Autodesk Inventor part; units mm, degrees
ref_plane "pins_to_body_XY" through (0, 0, 0) normal (0, -1, 0) x (1, 0, 0)
ref_plane "pins_to_body_YZ" through (0, 0, 0) normal (1, 0, 0) x (0, 0, 1)
ref_plane "pins_to_body_ZX" through (0, 0, 0) normal (0, 0, 1) x (0, -1, 0)
sketch "Sketch_1" plane through (0, 0, 0) normal (0, 1, 0) x (-1, 0, 0)
  line L0 (7.0485, -7.0485) -> (7.0485, 7.0485)
  line L1 (7.0485, 7.0485) -> (-7.0485, 7.0485)
  line L2 (-7.0485, 7.0485) -> (-7.0485, -7.0485)
  line L3 (-7.0485, -7.0485) -> (7.0485, -7.0485)
extrude "Extrusion1" add sketch "Sketch_1" along normal blind 0.0254
sketch "Sketch_3" plane through (0, 0, 7.0485) normal (0, 0, 1) x (1, 0, 0)
  line L0 (-0.7112, 0.0254) -> (-0.7112, -0.7366)
  line L1 (-0.7112, -0.7366) -> (-0.5842, -0.7366)
  line L2 (-0.5842, -0.7366) -> (-0.5842, -3.048)
  line L3 (-0.5842, -3.048) -> (-0.4318, -3.048)
  line L4 (-0.4318, -3.048) -> (-0.4318, -3.556)
  line L5 (-0.4318, -3.556) -> (-0.5842, -3.556)
  line L6 (-0.5842, -3.556) -> (-0.5842, -5.08)
  arc A0 (-0.5842, -5.08) -> (0.5842, -5.08) centre (0, -4.772) ccw
  line L7 (0.5842, -5.08) -> (0.5842, -3.556)
  line L8 (0.5842, -3.556) -> (0.4318, -3.556)
  line L9 (0.4318, -3.556) -> (0.4318, -3.048)
  line L10 (0.4318, -3.048) -> (0.5842, -3.048)
  line L11 (0.5842, -3.048) -> (0.5842, -0.7366)
  line L12 (0.5842, -0.7366) -> (0.7112, -0.7366)
  line L13 (0.7112, -0.7366) -> (0.7112, 0.0254)
  line L14 (0.7112, 0.0254) -> (-0.7112, 0.0254)
extrude "Extrusion2" add sketch "Sketch_3" against normal blind 0.6096
sketch "Sketch_5" plane through (0, 0, 0) normal (0, 0, 1) x (1, 0, 0)
  line L0 (4.0005, 0.0254) -> (4.0005, -3.2512)
  arc A0 (4.0005, -3.2512) -> (4.2545, -3.5052) centre (4.2545, -3.2512) ccw
  line L1 (4.2545, -3.5052) -> (5.7531, -3.5052)
  arc A1 (5.7531, -3.5052) -> (6.0071, -3.2512) centre (5.7531, -3.2512) ccw
  line L2 (6.0071, -3.2512) -> (6.0071, 0.0254)
  line L3 (6.0071, 0.0254) -> (4.0005, 0.0254)
  arc A2 (4.4577, -2.3876) -> (5.5499, -2.3876) centre (5.0038, -0.8728) ccw
  line L4 (5.5499, -2.3876) -> (5.5499, -0.5842)
  arc A3 (5.5499, -0.5842) -> (4.4577, -0.5842) centre (5.0038, -1.9147) ccw
  line L5 (4.4577, -0.5842) -> (4.4577, -2.3876)
extrude "Extrusion3" add sketch "Sketch_5" along normal mid plane 0.7874
sketch "Sketch_6" plane through (0, 0, 0) normal (0, 0, 1) x (1, 0, 0)
  line L0 (-6.0071, 0.0254) -> (-6.0071, -3.2512)
  arc A0 (-6.0071, -3.2512) -> (-5.7531, -3.5052) centre (-5.7531, -3.2512) ccw
  line L1 (-5.7531, -3.5052) -> (-4.2545, -3.5052)
  arc A1 (-4.2545, -3.5052) -> (-4.0005, -3.2512) centre (-4.2545, -3.2512) ccw
  line L2 (-4.0005, -3.2512) -> (-4.0005, 0.0254)
  line L3 (-4.0005, 0.0254) -> (-6.0071, 0.0254)
  line L4 (-5.5499, -0.5842) -> (-5.5499, -2.3876)
  arc A2 (-5.5499, -2.3876) -> (-4.4577, -2.3876) centre (-5.0038, -0.8728) ccw
  line L5 (-4.4577, -2.3876) -> (-4.4577, -0.5842)
  arc A3 (-4.4577, -0.5842) -> (-5.5499, -0.5842) centre (-5.0038, -1.9147) ccw
extrude "Extrusion4" add sketch "Sketch_6" along normal mid plane 0.7874
sketch "Sketch_7" plane through (0, 0, -4.699) normal (0, 0, 1) x (1, 0, 0)
  line L0 (4.0005, 0.0254) -> (4.0005, -2.7432)
  arc A0 (4.0005, -2.7432) -> (4.2545, -2.9972) centre (4.2545, -2.7432) ccw
  line L1 (4.2545, -2.9972) -> (5.7531, -2.9972)
  arc A1 (5.7531, -2.9972) -> (6.0071, -2.7432) centre (5.7531, -2.7432) ccw
  line L2 (6.0071, -2.7432) -> (6.0071, 0.0254)
  line L3 (6.0071, 0.0254) -> (4.0005, 0.0254)
  arc A2 (4.4577, -2.1336) -> (5.5499, -2.1336) centre (5.0038, -0.6188) ccw
  line L4 (5.5499, -2.1336) -> (5.5499, -0.3302)
  arc A3 (5.5499, -0.3302) -> (4.4577, -0.3302) centre (5.0038, -1.6607) ccw
  line L5 (4.4577, -0.3302) -> (4.4577, -2.1336)
extrude "Extrusion5" add sketch "Sketch_7" along normal mid plane 0.7874
sketch "Sketch_8" plane through (0, 0, -4.699) normal (0, 0, 1) x (1, 0, 0)
  line L0 (-6.0071, 0.0254) -> (-6.0071, -2.7432)
  arc A0 (-6.0071, -2.7432) -> (-5.7531, -2.9972) centre (-5.7531, -2.7432) ccw
  line L1 (-5.7531, -2.9972) -> (-4.2545, -2.9972)
  arc A1 (-4.2545, -2.9972) -> (-4.0005, -2.7432) centre (-4.2545, -2.7432) ccw
  line L2 (-4.0005, -2.7432) -> (-4.0005, 0.0254)
  line L3 (-4.0005, 0.0254) -> (-6.0071, 0.0254)
  line L4 (-5.5499, -0.3302) -> (-5.5499, -2.1336)
  arc A2 (-5.5499, -2.1336) -> (-4.4577, -2.1336) centre (-5.0038, -0.6188) ccw
  line L5 (-4.4577, -2.1336) -> (-4.4577, -0.3302)
  arc A3 (-4.4577, -0.3302) -> (-5.5499, -0.3302) centre (-5.0038, -1.6607) ccw
extrude "Extrusion6" add sketch "Sketch_8" along normal mid plane 0.7874
sketch "Sketch_9" plane through (0, 0, 4.699) normal (0, 0, 1) x (1, 0, 0)
  line L0 (4.0005, 0.0254) -> (4.0005, -2.7432)
  arc A0 (4.0005, -2.7432) -> (4.2545, -2.9972) centre (4.2545, -2.7432) ccw
  line L1 (4.2545, -2.9972) -> (5.7531, -2.9972)
  arc A1 (5.7531, -2.9972) -> (6.0071, -2.7432) centre (5.7531, -2.7432) ccw
  line L2 (6.0071, -2.7432) -> (6.0071, 0.0254)
  line L3 (6.0071, 0.0254) -> (4.0005, 0.0254)
  arc A2 (4.4577, -2.1336) -> (5.5499, -2.1336) centre (5.0038, -0.6188) ccw
  line L4 (5.5499, -2.1336) -> (5.5499, -0.3302)
  arc A3 (5.5499, -0.3302) -> (4.4577, -0.3302) centre (5.0038, -1.6607) ccw
  line L5 (4.4577, -0.3302) -> (4.4577, -2.1336)
extrude "Extrusion7" add sketch "Sketch_9" along normal mid plane 0.7874
sketch "Sketch_10" plane through (0, 0, 4.699) normal (0, 0, 1) x (1, 0, 0)
  line L0 (-6.0071, 0.0254) -> (-6.0071, -2.7432)
  arc A0 (-6.0071, -2.7432) -> (-5.7531, -2.9972) centre (-5.7531, -2.7432) ccw
  line L1 (-5.7531, -2.9972) -> (-4.2545, -2.9972)
  arc A1 (-4.2545, -2.9972) -> (-4.0005, -2.7432) centre (-4.2545, -2.7432) ccw
  line L2 (-4.0005, -2.7432) -> (-4.0005, 0.0254)
  line L3 (-4.0005, 0.0254) -> (-6.0071, 0.0254)
  line L4 (-5.5499, -0.3302) -> (-5.5499, -2.1336)
  arc A2 (-5.5499, -2.1336) -> (-4.4577, -2.1336) centre (-5.0038, -0.6188) ccw
  line L5 (-4.4577, -2.1336) -> (-4.4577, -0.3302)
  arc A3 (-4.4577, -0.3302) -> (-5.5499, -0.3302) centre (-5.0038, -1.6607) ccw
extrude "Extrusion8" add sketch "Sketch_10" along normal mid plane 0.7874
sketch "Sketch_4" plane through (0, 0, -7.0485) normal (0, 0, 1) x (1, 0, 0)
  line L0 (-0.7112, 0.0254) -> (-0.7112, -0.7366)
  line L1 (-0.7112, -0.7366) -> (-0.5842, -0.7366)
  line L2 (-0.5842, -0.7366) -> (-0.5842, -3.048)
  line L3 (-0.5842, -3.048) -> (-0.4318, -3.048)
  line L4 (-0.4318, -3.048) -> (-0.4318, -3.556)
  line L5 (-0.4318, -3.556) -> (-0.5842, -3.556)
  line L6 (-0.5842, -3.556) -> (-0.5842, -5.08)
  arc A0 (-0.5842, -5.08) -> (0.5842, -5.08) centre (0, -4.772) ccw
  line L7 (0.5842, -5.08) -> (0.5842, -3.556)
  line L8 (0.5842, -3.556) -> (0.4318, -3.556)
  line L9 (0.4318, -3.556) -> (0.4318, -3.048)
  line L10 (0.4318, -3.048) -> (0.5842, -3.048)
  line L11 (0.5842, -3.048) -> (0.5842, -0.7366)
  line L12 (0.5842, -0.7366) -> (0.7112, -0.7366)
  line L13 (0.7112, -0.7366) -> (0.7112, 0.0254)
  line L14 (0.7112, 0.0254) -> (-0.7112, 0.0254)
extrude "Extrusion9" add sketch "Sketch_4" along normal blind 0.6096
ref_plane "pins_to_body_XY" through (0, 0, 0) normal (0, -1, 0) x (1, 0, 0)
ref_plane "pins_to_body_YZ" through (0, 0, 0) normal (1, 0, 0) x (0, 0, 1)
ref_plane "pins_to_body_ZX" through (0, 0, 0) normal (0, 0, 1) x (0, -1, 0)
properties part number "tlD-pins"
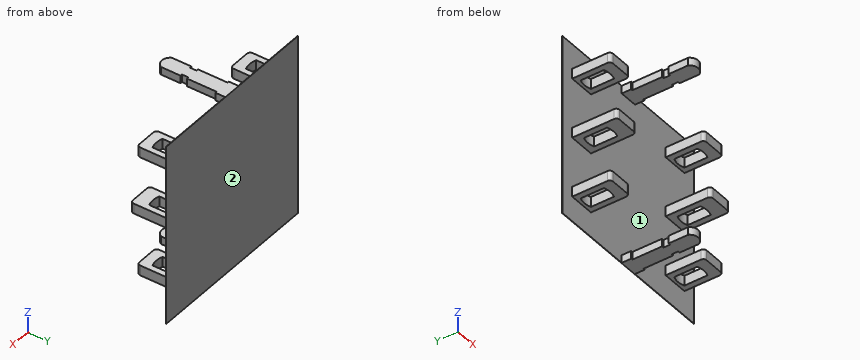
Part model, mm, in its own coordinate system. Face numbers are marked on the shaded views. Give positions to 0.01 mm unless a question says otherwise; leave off trailing zeros. Order: outer loops, then holes, each group sorted by start corner. A loop starts at its lowest first (then second) coordinate and runs counter-clockwise, first axis right, second up. Notation, with made-up numbers: M -12.5,22.5 L -0.5,22.5 A18 ccw -0.5,32.5 Z; hole C -1,33 d4. An arc over 180 degrees is marked long. Use a Markdown table: item, result. Add a question column.
(1) Saw through at A-A, the plane x = 4.75. Give the number of separate pieces and of enclosed holes in the cut face, and give its area (3 significant figures).
(2) Mould opens along Z. For the marked faces 1 and 2 say: +Z half, -Z half, draft (parallel to the pull), parting line (faces both ways), or undercut.
(3) Probe line 1 along X through (y, z) = (-3.75, 6.5); line 2 along X through (y, z) = (-2.8, -5). List the from-to ranges inside material, lowest first. Write a range as [from, to].
(4) Drop flat-ended pins along their axis: P1, Ø0.7, axis at y = -0.5, z = -6.5, coming from the -X side; P2, Ø3, axis at x = -3.5, y = -4.5, coming from the -Z side; P3, Ø1, axis at x = -0.5, z = -5, coming from the -Y side. Give the stop position or say it passes through.
(5) Saw through at B-B, the plane y = -4.45. Give the cut face in (x, z), and give its area (3 significant figures).
Answer key:
| question | item | result |
|---|---|---|
| 1 | separate pieces | 4 |
| 1 | enclosed holes | 0 |
| 1 | area | 3.20 mm^2 |
| 2 | face 1 | undercut |
| 2 | face 2 | draft |
| 3 | line 1 | [-0.58, 0.58] |
| 3 | line 2 | [-6, -4.01], [4.01, 6] |
| 4 | P1 | x = -0.71 |
| 4 | P2 | z = -0.39 |
| 4 | P3 | y = 0 |
| 5 | outline | M -0.58,-7.05 L 0.58,-7.05 L 0.58,-6.44 L -0.58,-6.44 Z; M -0.58,6.44 L 0.58,6.44 L 0.58,7.05 L -0.58,7.05 Z |
| 5 | area | 1.42 mm^2 |
